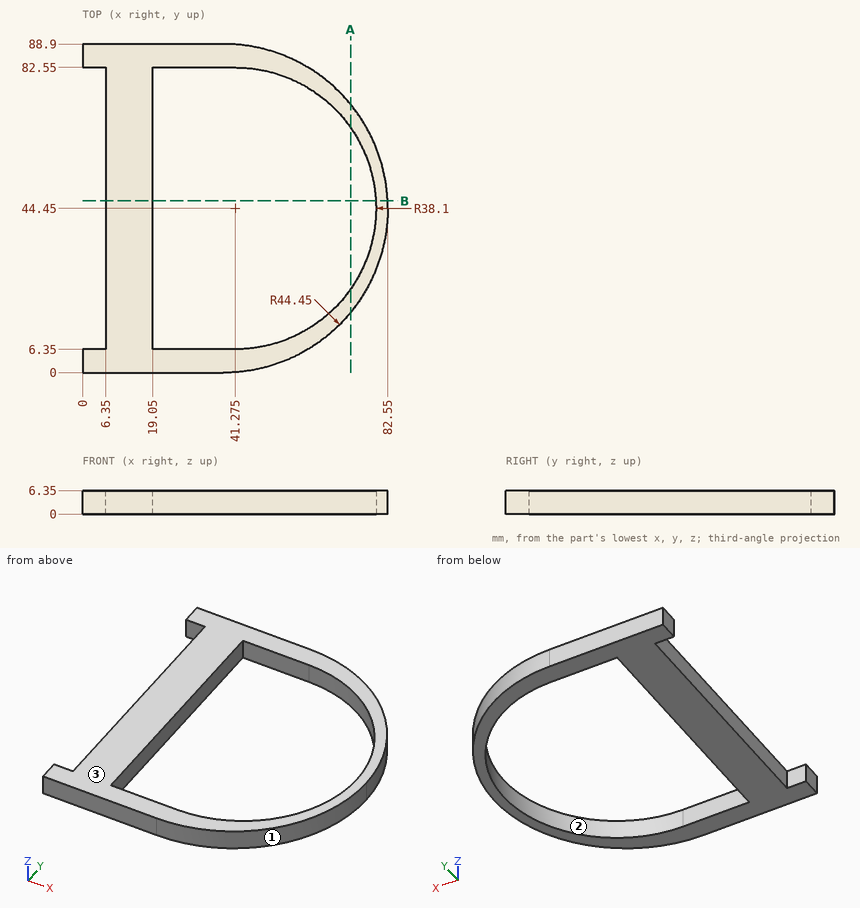
Geometry check sheet. Reference: drawing and pictorial views, mm from the part's lowest x, y, z. Give positions to 0.01 mm unless a question says otherwise; leave off trailing zeros. Write each loop counter-clockwise with the first axis right and the second up, starting at its lowest first coordinate (ties: lowest second). Pieces come first, ordered by that corner, then holes. Notation, with made-up numbers: M 33.25,88.5 L 40.25,88.5 A27 cw 40.25,105.5 Z; hole C 76.25,-7.75 d5. An arc over 180 degrees is marked long. Answer as CSV lines item,"result". Start each with the question number.
Q1. Section check B-B, the plane y = 46.5. Record the cut outline in (x, z), then the cut area to 3 significant figures.
Q2. Section check A-A, the plane x = 72.5. Record the cut outline in (y, z), then the cut area to 4 significant figures.
Q3. Material ranges on L1, parallel to Y at x = 23, z = 3; L2, parallel to X at y = 43.5, z = 4; L3, parallel to X at y = 35, z = 5, recorded low to high.
Q4. Go/stop test with flat-tipped pins: pin 1 (8 mm diameter, centred on x = 33, y = 13.5, fed in from -Z); pin 2 (3 mm diameter, centred on y = 52, z = 4, fed in from -X). Record where each tip stops, or that it passes through.
Q5. Release check for a two-part mould opening along Y. For the marked faces 1, 2 and 3 record: pulls with the +Y half, pulls with the -Y half, needs draft (parallel to the pull), parting line crosses it, or undercut.
Geometry says:
1,outline,"M 6.35,0 L 19.05,0 L 19.05,6.35 L 6.35,6.35 Z; M 79.32,0 L 82.5,0 L 82.5,6.35 L 79.32,6.35 Z"
1,area,"101 mm^2"
2,outline,"M 16.3,0 L 22.62,0 L 22.62,6.35 L 16.3,6.35 Z; M 66.28,0 L 72.6,0 L 72.6,6.35 L 66.28,6.35 Z"
2,area,"80.25 mm^2"
3,L1,"0 to 6.35, 82.55 to 88.9"
3,L2,"6.35 to 19.05, 79.36 to 82.54"
3,L3,"6.35 to 19.05, 78.18 to 81.53"
4,pin 1,"through"
4,pin 2,"x = 6.35"
5,face 1,"pulls with the -Y half"
5,face 2,"undercut"
5,face 3,"needs draft"
